The drawing under review shows one solid part. Ordinate dimensions are in mm from its lowest x, y, z. A direction names the side the tool comes from. Coordinates: 2 decimals unless noted, no trailing zeros. Write each loop counter-clockwise with the first axis right and the second up, starting at its lowest first coordinate (ties: lowest second). Pieces come first, ordered by that corner, then holes.
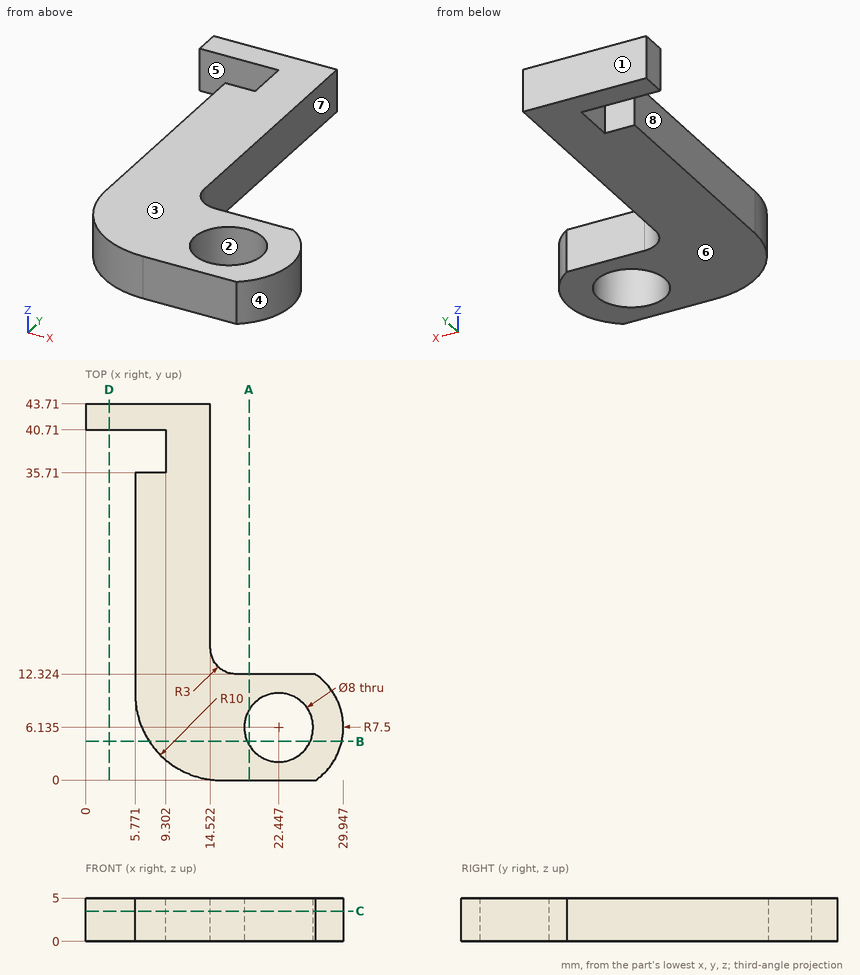
Q1. Add section B-B (y = 4.5). State the section outline as (x, z) points.
Ans:
outline: (7.42, 0) - (18.8, 0) - (18.8, 5) - (7.42, 5) - close; (26.1, 0) - (29.77, 0) - (29.77, 5) - (26.1, 5) - close
Q2. Add section A-A (x = 19). State the section outline as (y, z) points (1 decimal).
Ans:
outline: (0, 0) - (4.1, 0) - (4.1, 5) - (0, 5) - close; (8.2, 0) - (12.3, 0) - (12.3, 5) - (8.2, 5) - close
Q3. Tool access review of the marked faces 4, 5, 6, 7 and 8: name each direction out of +Z, -Z, +X, -X, +Y, -Y from which nothing blocks a thin tool from reaching the whole face with its end or side.
Ans:
face 4: +Z, -Z, +X
face 5: +Z, -Z, -X
face 6: -Z, +X, -X, +Y, -Y
face 7: +Z, -Z, +X, +Y
face 8: +Z, -Z, -X, -Y
Q4. Add section D-D (x = 2.75). State the section outline as (y, z) points, then the cut area to 3 significant figures.
Ans:
outline: (40.71, 0) - (43.71, 0) - (43.71, 5) - (40.71, 5) - close
area: 15.0 mm2
Q5. Clearance check with flat-ended pins moving along their axes: pin 1 Ø1 at (y, z) = (14.5, 2) entering from +X; pin 2 Ø1.5 at (x, z) = (20.5, 1.5) entering from +Y; pin 3 Ø2.5 at (y, z) = (36, 3) entering from +X. State where each tip first meets the part, or that it passes through.
Ans:
pin 1: stops at x = 14.83
pin 2: stops at y = 12.32
pin 3: stops at x = 14.52
Q6. Draft analysis for pull direction Y (two halves, no side actions). For the marked faces 1, 2 and 3, state which applies: +Y half, -Y half, draft (parallel to the pull), parting line (faces both ways), or undercut.
Ans:
face 1: +Y half
face 2: undercut
face 3: draft
Q7. Add section C-C (z = 3.5). State the section outline as (x, y) points (1 decimal).
Ans:
outline: (0, 40.7) - (9.3, 40.7) - (9.3, 35.7) - (5.8, 35.7) - (5.8, 10) arc R10 ccw to (15.8, 0) - (26.8, 0) arc R7.5 ccw to (26.7, 12.3) - (17.5, 12.3) arc R3 cw to (14.5, 15.3) - (14.5, 43.7) - (0, 43.7) - close; hole circle Ø8 at (22.4, 6.1)
Q8. For probe 1 along X at (y, z) = (34, 2.9); probe 2 along X at (y, z) = (8, 4.75) (1 decimal); probe 3 along Y at (x, z) = (19.25, 1.15) (1 decimal), list the stretches that pass through material, from the lowest coordinate up.
Ans:
probe 1: x = 5.77 to 14.52
probe 2: x = 6 to 18.9, 26 to 29.7
probe 3: y = 0 to 3.7, 8.5 to 12.3
